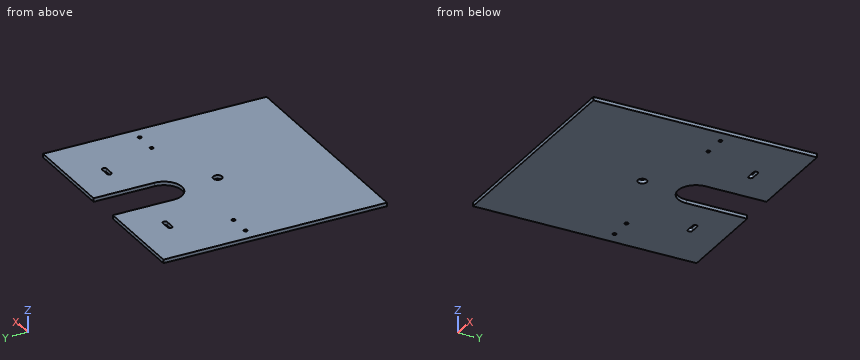
```python
from build123d import *

# Parameters (mm, degrees)
SKETCH1_W           = 250
SKETCH1_H           = 200
BOSS_EXTRUDE1_DEPTH = 4
SKETCH2_R           = 2
CUT_EXTRUDE1_DEPTH  = 4
SKETCH3_R           = 5
CUT_EXTRUDE2_DEPTH  = 4
SKETCH8_W           = 250
SKETCH8_H           = 4
BOSS_EXTRUDE2_DEPTH = 50


with BuildPart() as part:
    # Sketch1 → Boss-Extrude1 (new body)
    with BuildSketch(Plane.XY):
        Rectangle(SKETCH1_W, SKETCH1_H)
    extrude(amount=BOSS_EXTRUDE1_DEPTH)

    # Sketch2 → Cut-Extrude1 (cut)
    with BuildSketch(Plane.XY.offset(4)):
        with Locations((-110, 0)):
            Circle(SKETCH2_R)
        with Locations((-85, 0)):
            Circle(SKETCH2_R)
        with Locations((110, 0)):
            Circle(SKETCH2_R)
        with Locations((85, 0)):
            Circle(SKETCH2_R)
    extrude(amount=-CUT_EXTRUDE1_DEPTH, mode=Mode.SUBTRACT)

    # Sketch3 → Cut-Extrude2 (cut)
    with BuildSketch(Plane.XY.offset(4)):
        with Locations((0, -28)):
            Circle(SKETCH3_R)
        with BuildLine():
            Line((20, 32), (20, 100))
            Line((20, 100), (-20, 100))
            Line((-20, 100), (-20, 32))
            ThreePointArc((-20, 32), (0, 12), (20, 32))
        make_face()
        with BuildLine():
            Line((-68, 64.5), (-58, 64.5))
            ThreePointArc((-58, 64.5), (-55.5, 62), (-58, 59.5))
            Line((-58, 59.5), (-68, 59.5))
            ThreePointArc((-68, 59.5), (-70.5, 62), (-68, 64.5))
        make_face()
        with BuildLine():
            Line((58, 59.5), (68, 59.5))
            ThreePointArc((68, 59.5), (70.5, 62), (68, 64.5))
            Line((68, 64.5), (58, 64.5))
            ThreePointArc((58, 64.5), (55.5, 62), (58, 59.5))
        make_face()
    extrude(amount=-CUT_EXTRUDE2_DEPTH, mode=Mode.SUBTRACT)

    # Sketch8 → Boss-Extrude2 (add)
    with BuildSketch(Plane.XZ.offset(100)):
        with Locations((0, 2)):
            Rectangle(SKETCH8_W, SKETCH8_H)
    extrude(amount=BOSS_EXTRUDE2_DEPTH)


solid = part.part
```
Design review of the part built by this model. Coordinates are the model's own, in mm. Coordinates: 2 decimals unless noted, no trailing zeros. Write each loop counter-clockwise with the first axis right and the second up, starting at its lowest first coordinate (ties: lowest second). Pieces come first, ordered by that corner, then holes. Notation, with made-up numbers: M 71,34 L 127,34 A33 cw 127,70 Z; hole C 28,-4 d6. An arc over 180 degrees is marked long. Answer as a JSON object with one key per item and string values.
Item 1: Add section A-A, the plane x = 0. Give the boundary of the cut face in (y, z).
Outcome:
{"outline": "M -150,0 L -33,0 L -33,4 L -150,4 Z; M -23,0 L 12,0 L 12,4 L -23,4 Z"}
Item 2: Add section B-B, the plane y = 76.5. Give the boundary of the cut face in (x, z).
Outcome:
{"outline": "M -125,0 L -20,0 L -20,4 L -125,4 Z; M 20,0 L 125,0 L 125,4 L 20,4 Z"}
Item 3: Wall thickness on probe 1 along Y at (x, z) = (110, 1.7); probe 2 along X at (y, z) = (86.5, 3.65); probe 3 along Y at (x, z) = (58, 3.3): over which ranges is each line inside the solid? List them lowest first.
Outcome:
{"probe 1": "-150 to -2, 2 to 100", "probe 2": "-125 to -20, 20 to 125", "probe 3": "-150 to 59.5, 64.5 to 100"}
Item 4: Insertion check: pin 1 Ø4 at (x, y) = (44, -38.5) entering from -Z. The pin has a flat end and moves straight along its axis. Give the tip position at first contact, or say it passes through.
Outcome:
{"pin 1": "z = 0"}
Item 5: Add section C-C, the plane z = 0.7. Give the boundary of the cut face in (x, y), and give its area (3 significant figures).
Outcome:
{"outline": "M -125,-150 L 125,-150 L 125,100 L 20,100 L 20,32 A20 cw -20,32 L -20,100 L -125,100 Z; hole C -110,0 d4; hole C -85,0 d4; hole M -68,59.5 L -58,59.5 A2.5 ccw -58,64.5 L -68,64.5 A2.5 ccw Z; hole C 0,-28 d10; hole M 58,59.5 L 68,59.5 A2.5 ccw 68,64.5 L 58,64.5 A2.5 ccw Z; hole C 85,0 d4; hole C 110,0 d4", "area": "58,900 mm²"}
